```python
from build123d import *

# Parameters (mm, degrees)
SKETCH_1_W               = 22
SKETCH_1_H               = 21
EXTRUDE_1_DEPTH          = 2.86
EXTRUDE_2_DEPTH          = 22
CUT_EXTRUDE_1_DEPTH      = 16.724185194
CUT_EXTRUDE_1_DEPTH_BACK = 16.724185194
SKETCH_3_R               = 1.7


with BuildPart() as part:
    # 草图1 → 凸台-拉伸1 (new body)
    with BuildSketch(Plane.XY):
        Rectangle(SKETCH_1_W, SKETCH_1_H)
    extrude(amount=EXTRUDE_1_DEPTH)

    # 草图2 → 凸台-拉伸2 (add)
    with BuildSketch(Plane(origin=(11, 0, 0), x_dir=(0, 0, -1), z_dir=(1, 0, 0))):
        Polygon((1.14, -10.158179307), (0, -9.5), (0, -10.5), (1.14, -10.5), align=None)
        Polygon((1.14, -5.158179307), (0, -4.5), (0, -7.316358614), (1.14, -6.658179307), align=None)
        Polygon((1.14, -0.158179307), (0, 0.5), (0, -2.316358614), (1.14, -1.658179307), align=None)
        Polygon((1.14, 4.841820693), (0, 5.5), (0, 2.683641386), (1.14, 3.341820693), align=None)
        Polygon((1.14, 9.841820693), (0, 10.5), (0, 7.683641386), (1.14, 8.341820693), align=None)
    extrude(amount=-EXTRUDE_2_DEPTH)

    # 草图3 → 切除-拉伸1 (cut, two sides: drawn at the far end of the back side and taken through both)
    with BuildSketch(Plane.XY.offset(2.86).offset(-CUT_EXTRUDE_1_DEPTH_BACK)):
        with Locations(Location((7.5, 7.5, 0), (0, 0, 6.201440198))):
            Circle(SKETCH_3_R)
        with Locations(Location((7.5, -7.5, 0), (0, 0, 6.201440198))):
            Circle(SKETCH_3_R)
        with Locations(Location((-7.5, -7.5, 0), (0, 0, 6.201440198))):
            Circle(SKETCH_3_R)
        with Locations(Location((-7.5, 7.5, 0), (0, 0, 6.201440198))):
            Circle(SKETCH_3_R)
    extrude(amount=CUT_EXTRUDE_1_DEPTH + CUT_EXTRUDE_1_DEPTH_BACK, mode=Mode.SUBTRACT)


solid = part.part
```
The listing builds one solid part. Answer for the finished solid, in the listing's coordinates (mm). A direction names the side the tool comes from. Round coordinates to 2 decimals unless told otherwise and drop trailing zeros. Write each loop counter-clockwise with the first axis right and the second up, starting at its lowest first coordinate (ties: lowest second). Pieces come first, ordered by that corner, then holes. Notation, with made-up numbers: (-10, -36) -> (42, -36) arc R7 ccw to (42, -32) -> close; hole circle Ø11 at (-27, -19.5). An arc over 180 degrees is marked (long way). Answer as a JSON object with one key per item and string values. Group by question number.
Q1. Section B-B (z = -0.5) is taken. Write down the section's boundary in (x, y).
Q2. Straight lines are drawn through the part: line 1 along X through (y, z) = (-7.5, 1.8); line 2 along Y through (x, z) = (-7.5, 1.9); line 3 along Y through (x, z) = (5.25, -0.85). For each, find the intervals that lie inside material, in ascending order.
Q3. Section A-A (x = -7.5) is taken. Write down the section's boundary in (y, z), plus the area to 3 significant figures.
Q4. Which of the six approach directions +Z, -Z, +X, -X, +Y, -Y give full straight-line access (tool end or side, diameter ignored) to faces 4 (the face through (0.154, 5.166, -0.578)), 5 (the face through (0, -1, -1.14))?
Q5. Section D-D (x = 0.25) is taken. Write down the section's boundary in (y, z), plus the area to 3 significant figures.
Q6. Determine the mould class of faces 1 (the face through (7.098, 9.152, 1.276)), 2 (the face through (11, 0, 1)), 3 (the face through (0, -8, 0)) for opening direction X: pulls with the +X half, pulls with the -X half, needs draft (parallel to the pull), parting line crosses it, or undercut.
Q7. Section C-C (y = 8) is taken. Write down the section's boundary in (x, z).
Q8. Each of these flat-tipped pins is pushed along its axis until it touches: pin 1 Ø1.7 at (x, y) = (-0.5, -3) entering from -Z; pin 2 Ø0.7 at (x, y) = (-3, -8) entering from -Z; pin 3 Ø3 at (x, y) = (-7.5, 7) entering from +Z. Where does it stop, or does it pass through?
Check values:
{
 "1": {"outline": "(-11, -10.5) -> (11, -10.5) -> (11, -9.79) -> (-11, -9.79) -> close; (-11, -7.03) -> (-9.13, -7.03) arc R1.7 cw to (-5.87, -7.03) -> (5.87, -7.03) arc R1.7 cw to (9.13, -7.03) -> (11, -7.03) -> (11, -4.79) -> (-11, -4.79) -> close; (-11, -2.03) -> (11, -2.03) -> (11, 0.21) -> (-11, 0.21) -> close; (-11, 2.97) -> (11, 2.97) -> (11, 5.21) -> (-11, 5.21) -> close; (-11, 7.97) -> (-9.13, 7.97) arc R1.7 cw to (-5.87, 7.97) -> (5.87, 7.97) arc R1.7 cw to (9.13, 7.97) -> (11, 7.97) -> (11, 10.21) -> (-11, 10.21) -> close"},
 "2": {"line 1": "-11 to -9.2, -5.8 to 5.8, 9.2 to 11", "line 2": "-10.5 to -9.2, -5.8 to 5.8, 9.2 to 10.5", "line 3": "-10.5 to -9.99, -6.83 to -4.99, -1.83 to 0.01, 3.17 to 5.01, 8.17 to 10.01"},
 "3": {"outline": "(-10.5, -1.14) -> (-10.16, -1.14) -> (-9.5, 0) -> (-9.2, 0) -> (-9.2, 2.86) -> (-10.5, 2.86) -> close; (-5.8, -1.14) -> (-5.16, -1.14) -> (-4.5, 0) -> (-2.32, 0) -> (-1.66, -1.14) -> (-0.16, -1.14) -> (0.5, 0) -> (2.68, 0) -> (3.34, -1.14) -> (4.84, -1.14) -> (5.5, 0) -> (5.8, 0) -> (5.8, 2.86) -> (-5.8, 2.86) -> close; (9.2, -1.14) -> (9.84, -1.14) -> (10.5, 0) -> (10.5, 2.86) -> (9.2, 2.86) -> close", "area": "48.5 mm^2"},
 "4": {"face 4": "-Z, +X, -X", "face 5": "-Z, +X, -X, +Y, -Y"},
 "5": {"outline": "(-10.5, -1.14) -> (-10.16, -1.14) -> (-9.5, 0) -> (-7.32, 0) -> (-6.66, -1.14) -> (-5.16, -1.14) -> (-4.5, 0) -> (-2.32, 0) -> (-1.66, -1.14) -> (-0.16, -1.14) -> (0.5, 0) -> (2.68, 0) -> (3.34, -1.14) -> (4.84, -1.14) -> (5.5, 0) -> (7.68, 0) -> (8.34, -1.14) -> (9.84, -1.14) -> (10.5, 0) -> (10.5, 2.86) -> (-10.5, 2.86) -> close", "area": "70.7 mm^2"},
 "6": {"face 1": "undercut", "face 2": "pulls with the +X half", "face 3": "needs draft"},
 "7": {"outline": "(-11, -0.55) -> (-9.12, -0.55) -> (-9.12, 2.86) -> (-11, 2.86) -> close; (-5.88, -0.55) -> (5.88, -0.55) -> (5.88, 2.86) -> (-5.88, 2.86) -> close; (9.12, -0.55) -> (11, -0.55) -> (11, 2.86) -> (9.12, 2.86) -> close"},
 "8": {"pin 1": "z = -0.29", "pin 2": "z = 0", "pin 3": "z = 2.86"}
}
